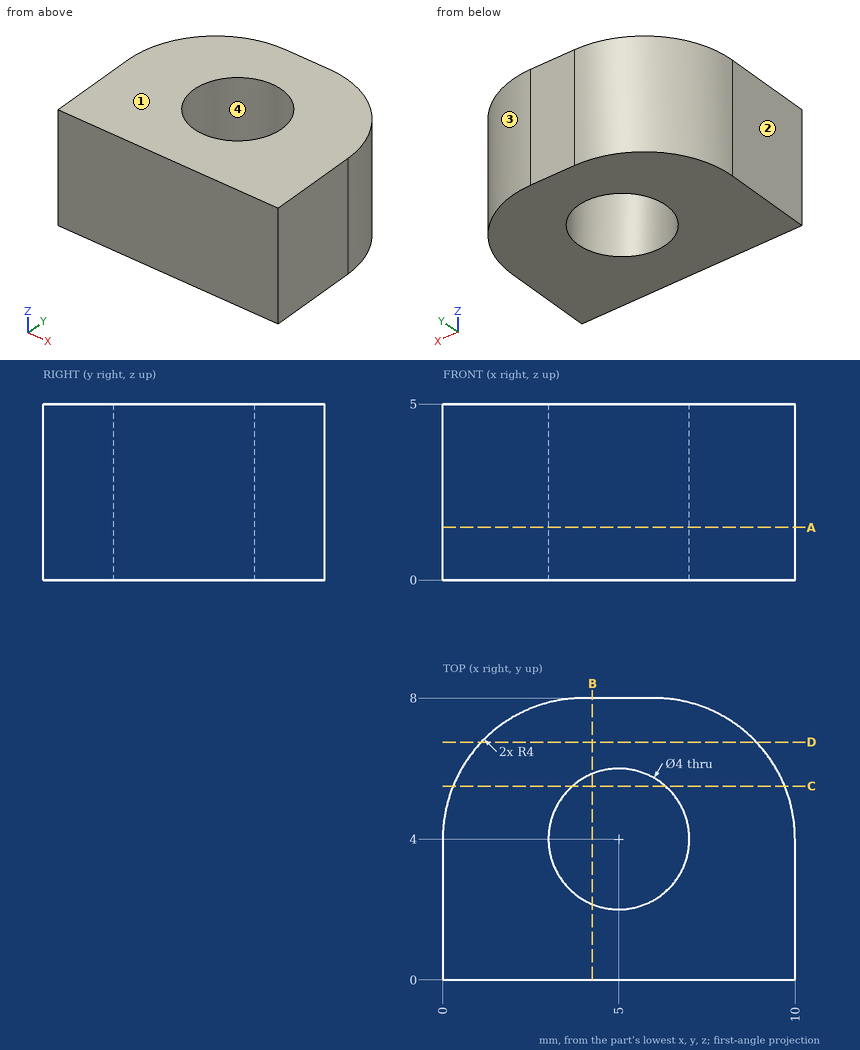
Study the drawing (mm; zero at the part's minimum x, y, z) and answer. Coordinates: 2 decimals unless noted, no trailing zeros. Order: outer loops, then holes, each group sorted by start corner. A loop starts at its lowest first (then second) coordinate and runs counter-clockwise, first axis right, second up. Notation, with made-up numbers: M -4.75,-22.5 L 16.25,-22.5 A13 cw 16.25,-3.5 Z; hole C 77.25,79.25 d8. An arc over 180 degrees is marked long. Use CSV: the item, a comma, the result in double quotes.
Q1. Determine the mould class of the marked faces 1, 2, 3 and 4 for opening direction X: pulls with the +X half, pulls with the -X half, needs draft (parallel to the pull), parting line crosses it, or undercut.
Here are the results:
face 1,"needs draft"
face 2,"pulls with the -X half"
face 3,"pulls with the +X half"
face 4,"undercut"
Q2. Section A-A (z = 1.5) is taken. Determine the outline of the cut face in (x, y).
Here are the results:
outline,"M 0,0 L 10,0 L 10,4 A4 ccw 6,8 L 4,8 A4 ccw 0,4 Z; hole C 5,4 d4"
Q3. Section D-D (y = 6.75) is taken. Determine the outline of the cut face in (x, z), then the cut area to 3 significant figures.
Here are the results:
outline,"M 1.1,0 L 8.9,0 L 8.9,5 L 1.1,5 Z"
area,"39.0 mm2"
Q4. Section C-C (y = 5.5) is taken. Determine the outline of the cut face in (x, z).
Here are the results:
outline,"M 0.29,0 L 3.68,0 L 3.68,5 L 0.29,5 Z; M 6.32,0 L 9.71,0 L 9.71,5 L 6.32,5 Z"
Q5. Section B-B (x = 4.25) is taken. Determine the outline of the cut face in (y, z).
Here are the results:
outline,"M 0,0 L 2.15,0 L 2.15,5 L 0,5 Z; M 5.85,0 L 8,0 L 8,5 L 5.85,5 Z"
Q6. Given pin 1 Ø1 at (x, y) = (3, 7) entering from -Z; pin 2 Ø1 at (y, z) = (7, 2) entering from +X, each flat-ended and moving along its own axis, determine where each tip first touches the part or whether it passes through.
Here are the results:
pin 1,"z = 0"
pin 2,"x = 9.12"
Q7. Straight lines are drawn through the part: L1, parallel to Y at x = 5, z = 1.35; L2, parallel to Y at x = 5.75, z = 4.15; L3, parallel to X at y = 6.5, z = 3.05. For each, find the intervals that lie inside material, in ascending order.
Here are the results:
L1,"0 to 2, 6 to 8"
L2,"0 to 2.15, 5.85 to 8"
L3,"0.88 to 9.12"
